Could you check a few things on this model? Use its own coordinates, in mm. Give positions to 0.01 mm unless a question says otherwise; leave off trailing zeros. Write each loop counter-clockwise with the first axis right and the second up, starting at its lowest first coordinate (ties: lowest second). Pieces come first, ordered by that corner, then holes. Notation, with made-up numbers: (54.5, -8.5) - (63.5, -8.5) arc R8 cw to (63.5, -2.5) - close; hole circle Ø10 at (-25, 87.5). An arc over 180 degrees is marked (long way). Use one line per item in the form item = value.
```python
from build123d import *

# Parameters (mm, degrees)
F1_DEPTH = 88.9
F2_W     = 88.9
F2_H     = 19.05
F3_DEPTH = 6.35


with BuildPart() as f1:
    # F0 (on Front) → F1 (new body, symmetric)
    with BuildSketch(Plane.XZ):
        Polygon((19.05, 514.35), (19.05, 19.05), (38.1, 0), (38.1, 533.4), align=None)
    extrude(amount=F1_DEPTH, both=True)

    # F2 (on face) → F3 (cut)
    with BuildSketch(Plane(origin=(19.05, 0, 0), x_dir=(0, -1, 0), z_dir=(-1, 0, 0))):
        with Locations((-44.45, 180.975)):
            Rectangle(F2_W, F2_H)
        with Locations((-44.45, 352.425)):
            Rectangle(F2_W, F2_H)
    extrude(amount=-F3_DEPTH, mode=Mode.SUBTRACT)


solid = f1.part
```
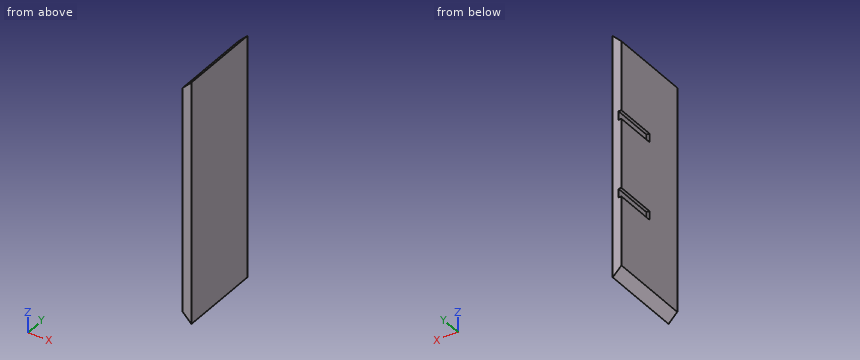
1. For pin 1 (1.5 mm diameter, centred on x = 33.5, y = 71, fed in from -Z); pin 2 (1.9 mm diameter, centred on x = 22.5, z = 183, fed in from +Y); pin 3 (7 mm diameter, centred on x = 22.5, y = 64, fed in from -Z), each with a flat end and sliding along its axis, tell me the tip position at first contact or that it passes through.
Response values:
pin_1 = 3.85
pin_2 = 0
pin_3 = 12.1
2. Imagine slicing it at C-C, the plane y = -66.5. List the corners of the cut face in (x, z) for me, and give its area (3 significant figures).
Response values:
outline = (19.05, 19.05) - (38.1, 0) - (38.1, 533.4) - (19.05, 514.35) - close
area = 9,800 mm²
3. Imagine slicing it at A-A, the plane y = 49. List the corners of the cut face in (x, z) for me, and give its area (3 significant figures).
Response values:
outline = (19.05, 19.05) - (38.1, 0) - (38.1, 533.4) - (19.05, 514.35) - (19.05, 361.95) - (25.4, 361.95) - (25.4, 342.9) - (19.05, 342.9) - (19.05, 190.5) - (25.4, 190.5) - (25.4, 171.45) - (19.05, 171.45) - close
area = 9,560 mm²
4. Imagine slicing it at B-B, the plane x = 28.5. List the corners of the cut face in (y, z) for me.
Response values:
outline = (-88.9, 9.6) - (88.9, 9.6) - (88.9, 523.8) - (-88.9, 523.8) - close
5. If I drill on line 1 (Z direction, x = 23.75, y = 70); line 2 (Z direction, x = 21.25, y = 18.5); line 3 (Z direction, x = 28.5, y = -72.5), over which ranges is the centre line in solid material (lowest first)? Write a range as from..to.
Response values:
line_1 = 14.35..171.45, 190.5..342.9, 361.95..519.05
line_2 = 16.85..171.45, 190.5..342.9, 361.95..516.55
line_3 = 9.6..523.8
